```python
from build123d import *

# Parameters (mm, degrees)
F0_W     = 5
F0_H     = 5
F1_DEPTH = 10


with BuildPart() as f1:
    # F0 (on Top) → F1 (new body)
    with BuildSketch(Plane.XY):
        with BuildLine():
            Line((2.5, -2.5), (73.9577582137, -2.5))
            ThreePointArc((73.9577582137, -2.5), (73.9894387998, -1.2501784241), (74, 0))
            ThreePointArc((74, 0), (73.9894387998, 1.2501784241), (73.9577582137, 2.5))
            Line((73.9577582137, 2.5), (2.5, 2.5))
            Line((2.5, 2.5), (2.5, -2.5))
        make_face()
        with BuildLine():
            Line((-2.5, 2.5), (2.5, 2.5))
            Line((2.5, 2.5), (2.5, 73.9577582137))
            ThreePointArc((2.5, 73.9577582137), (0, 74), (-2.5, 73.9577582137))
            Line((-2.5, 73.9577582137), (-2.5, 2.5))
        make_face()
        with BuildLine():
            ThreePointArc((-2.5, -73.9577582137), (0, -74), (2.5, -73.9577582137))
            Line((2.5, -73.9577582137), (2.5, -2.5))
            Line((2.5, -2.5), (-2.5, -2.5))
            Line((-2.5, -2.5), (-2.5, -73.9577582137))
        make_face()
        with BuildLine():
            Line((-75, 2.5), (-75, -2.5))
            Line((-75, -2.5), (-73.9577582137, -2.5))
            ThreePointArc((-73.9577582137, -2.5), (-74, 0), (-73.9577582137, 2.5))
            Line((-73.9577582137, 2.5), (-75, 2.5))
        make_face()
        with BuildLine():
            Line((2.5, 73.9577582137), (2.5, 75))
            Line((2.5, 75), (-2.5, 75))
            Line((-2.5, 75), (-2.5, 73.9577582137))
            ThreePointArc((-2.5, 73.9577582137), (0, 74), (2.5, 73.9577582137))
        make_face()
        with BuildLine():
            Line((-2.5, -75), (2.5, -75))
            Line((2.5, -75), (2.5, -73.9577582137))
            ThreePointArc((2.5, -73.9577582137), (0, -74), (-2.5, -73.9577582137))
            Line((-2.5, -73.9577582137), (-2.5, -75))
        make_face()
        with BuildLine():
            Line((-73.9577582137, -2.5), (-2.5, -2.5))
            Line((-2.5, -2.5), (-2.5, 2.5))
            Line((-2.5, 2.5), (-73.9577582137, 2.5))
            ThreePointArc((-73.9577582137, 2.5), (-74, 0), (-73.9577582137, -2.5))
        make_face()
        with BuildLine():
            Line((73.9577582137, -2.5), (75, -2.5))
            Line((75, -2.5), (75, 2.5))
            Line((75, 2.5), (73.9577582137, 2.5))
            ThreePointArc((73.9577582137, 2.5), (73.9894387998, 1.2501784241), (74, 0))
            ThreePointArc((74, 0), (73.9894387998, -1.2501784241), (73.9577582137, -2.5))
        make_face()
        Rectangle(F0_W, F0_H)
        with BuildLine():
            Line((-75, -75), (-2.5, -75))
            Line((-2.5, -75), (-2.5, -73.9577582137))
            ThreePointArc((-2.5, -73.9577582137), (-52.3259018078, -52.3259018078), (-73.9577582137, -2.5))
            Line((-73.9577582137, -2.5), (-75, -2.5))
            Line((-75, -2.5), (-75, -75))
        make_face()
        with BuildLine():
            Line((2.5, -75), (75, -75))
            Line((75, -75), (75, -2.5))
            Line((75, -2.5), (73.9577582137, -2.5))
            ThreePointArc((73.9577582137, -2.5), (52.3259018078, -52.3259018078), (2.5, -73.9577582137))
            Line((2.5, -73.9577582137), (2.5, -75))
        make_face()
        with BuildLine():
            Line((-75, 75), (-75, 2.5))
            Line((-75, 2.5), (-73.9577582137, 2.5))
            ThreePointArc((-73.9577582137, 2.5), (-52.3259018078, 52.3259018078), (-2.5, 73.9577582137))
            Line((-2.5, 73.9577582137), (-2.5, 75))
            Line((-2.5, 75), (-75, 75))
        make_face()
        with BuildLine():
            Line((73.9577582137, 2.5), (75, 2.5))
            Line((75, 2.5), (75, 75))
            Line((75, 75), (2.5, 75))
            Line((2.5, 75), (2.5, 73.9577582137))
            ThreePointArc((2.5, 73.9577582137), (52.3259018078, 52.3259018078), (73.9577582137, 2.5))
        make_face()
    extrude(amount=F1_DEPTH)


solid = f1.part
```
Can you work these out from the model? Positions are in its coordinate system, mm. A direction names the side the tool comes from. Coordinates: 2 decimals unless noted, no trailing zeros. Write each loop counter-clockwise with the first axis right and the second up, starting at its lowest first coordinate (ties: lowest second). Pieces come first, ordered by that corner, then holes. Notation, with made-up numbers: M 25,10 L 43,10 A23 ccw 43,24 Z; hole C 63.25,10 d6. An arc over 180 degrees is marked long. Answer as CSV lines item,"result".
Item 1: Imagine slicing it at B-B on x = -18.5. List the corners of the cut face in (y, z) for me, plus the area to 3 significant figures.
Geometry results:
outline,"M -75,0 L -71.65,0 L -71.65,10 L -75,10 Z; M -2.5,0 L 2.5,0 L 2.5,10 L -2.5,10 Z; M 71.65,0 L 75,0 L 75,10 L 71.65,10 Z"
area,"117 mm2"
Item 2: Please list where these lines run through material, in increasing order: line 1 along Y through (x, z) = (-32, 1); line 2 along X through (y, z) = (-9.5, 3); line 3 along X through (y, z) = (-4, 9.25).
Geometry results:
line 1,"y = -75 to -66.72, -2.5 to 2.5, 66.72 to 75"
line 2,"x = -75 to -73.39, -2.5 to 2.5, 73.39 to 75"
line 3,"x = -75 to -73.89, -2.5 to 2.5, 73.89 to 75"
Item 3: On a 3-axis mill with a long thin cutter (end or side, diameter ignored), from which of +Z, -Z, +X, -X, +Y, -Y can I reach the whole of each face in a straight line? I mean faces 4 (the flat face through (75, -1, 5)), 5 (the flat face through (-38, 2.5, 5)). Say none if no direction works.
Geometry results:
face 4,"+Z, -Z, +X, +Y, -Y"
face 5,"+Z, -Z"
Item 4: We'd pull the mould along Y, two halves only. Please class faces 1 (the flat face through (-1, 1, 0)), 2 (the flat face through (-2.5, -38, 5)), 3 (the flat face through (1, 75, 5)): +Y half, -Y half, draft (parallel to the pull), parting line (faces both ways), or undercut.
Geometry results:
face 1,"draft"
face 2,"undercut"
face 3,"+Y half"
Item 5: Imagine slicing it at A-A on y = -53. List the corners of the cut face in (x, z) for me.
Geometry results:
outline,"M -75,0 L -51.64,0 L -51.64,10 L -75,10 Z; M -2.5,0 L 2.5,0 L 2.5,10 L -2.5,10 Z; M 51.64,0 L 75,0 L 75,10 L 51.64,10 Z"
Item 6: Imagine slicing it at C-C on z = 5.75. List the corners of the cut face in (x, y) for me.
Geometry results:
outline,"M -75,-75 L 75,-75 L 75,75 L -75,75 Z; hole M -73.96,-2.5 A74 ccw -2.5,-73.96 L -2.5,-2.5 Z; hole M -73.96,2.5 L -2.5,2.5 L -2.5,73.96 A74 ccw Z; hole M 2.5,-73.96 A74 ccw 73.96,-2.5 L 2.5,-2.5 Z; hole M 2.5,2.5 L 73.96,2.5 A74 ccw 2.5,73.96 Z"
